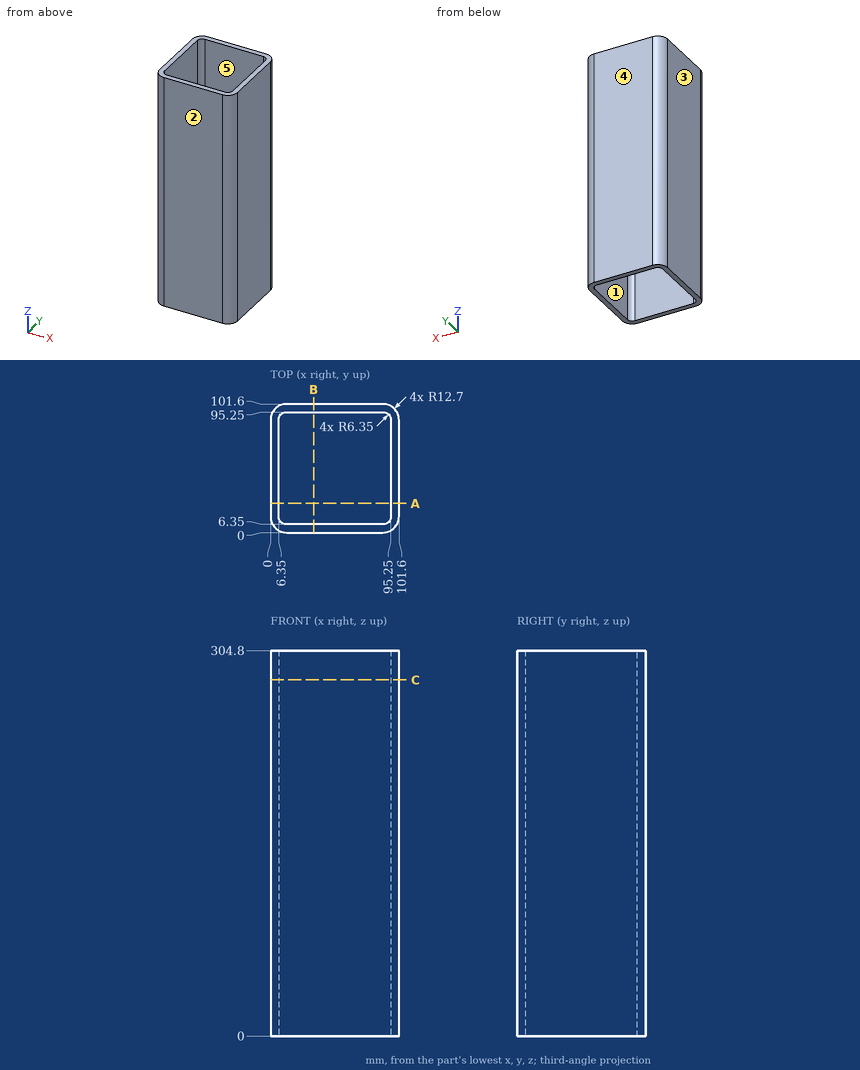
Study the drawing (mm; zero at the part's minimum x, y, z) and answer. A direction names the side the tool comes from. Give positions to 0.01 mm unless a question says otherwise; leave off trailing zeros. Order: outer loops, then holes, each group sorted by start corner. A loop starts at its lowest first (then second) coordinate and runs counter-clockwise, first axis right, second up. Notation, with made-up numbers: M 61,-39 L 97,-39 A19 ccw 97,-4 Z; hole C 49.25,-29 d7. An arc over 180 degrees is marked long. Put each result on its own line as item: value. Start each with the question number.
Item 1: Which of the six approach directions +Z, -Z, +X, -X, +Y, -Y give full straight-line access (tool end or side, diameter ignored) to the marked faces 4 and 5?
Item 2: For a pull along X with two mould halves and no side action, classify the marked faces 1, 2 and 3 as +X half, -X half, draft (parallel to the pull), parting line (faces both ways), or undercut.
Item 3: The part is cut by section A-A, the plane y = 23. Determine the outline of the cut face in (x, z).
Item 4: The part is cut by section C-C, the plane z = 281.5. Determine the outline of the cut face in (x, y), and give its area (3 significant figures).
Item 5: Find the intervals of material crossed by line 1 along X through (y, z) = (53.5, 143.5); line 2 along Y through (x, z) = (93, 178), in increasing order.
Answer key:
1. face 4: +Z, -Z, +X, -X, +Y
1. face 5: +Z, -Z
2. face 1: undercut
2. face 2: draft
2. face 3: -X half
3. outline: M 0,0 L 6.35,0 L 6.35,304.8 L 0,304.8 Z; M 95.25,0 L 101.6,0 L 101.6,304.8 L 95.25,304.8 Z
4. outline: M 0,12.7 A12.7 ccw 12.7,0 L 88.9,0 A12.7 ccw 101.6,12.7 L 101.6,88.9 A12.7 ccw 88.9,101.6 L 12.7,101.6 A12.7 ccw 0,88.9 Z; hole M 6.35,12.7 A6.35 ccw 12.7,6.35 L 88.9,6.35 A6.35 ccw 95.25,12.7 L 95.25,88.9 A6.35 ccw 88.9,95.25 L 12.7,95.25 A6.35 ccw 6.35,88.9 Z
4. area: 2,320 mm²
5. line 1: x = 0 to 6.35, 95.25 to 101.6
5. line 2: y = 0.68 to 7.85, 93.75 to 100.92
